Design review of the part built by this model. Coordinates are the model's own, in mm. Face numbers are marked on the shaded views. A direction names the side the tool comes from. Give positions to 0.01 mm unless a question says otherwise; leave off trailing zeros. Loops run counter-clockwise (first coordinate to the right, second up) from the corner with the lowest first, then second, coordinate; pieces in that order, holes last. Notation, with made-up numbers: (-10.75, 24) - (26.25, 24) arc R12 ccw to (26.25, 41) - close; hole circle Ø4 at (46.5, 75). An arc over 180 degrees is marked (long way). Write each question's results on one line, items separated by ' | '.
from build123d import *

# Parameters (mm, degrees)
BASE_DEPTH                = 7
SKETCH2_W                 = 9.8
SKETCH2_H                 = 13.6
PCB_CUTOUT_DEPTH          = 2.5
BASKET_WIRE_GROOVES_DEPTH = 30.49321956
SKETCH5_R                 = 1.4
SCREW_HOLES_DEPTH         = 28.14498112
F_1MM_EDGE_FILLETS_R      = 1


with BuildPart() as part:
    # Sketch1 → Base (new body)
    with BuildSketch(Plane(origin=(0, 0, 0), x_dir=(1, 0, 0), z_dir=(0, 1, 0))):
        Polygon((-8.9, 10.8), (-8.9, 5), (-23.9, 5), (-23.9, -5), (-8.9, -5), (-8.9, -10.8), (8.9, -10.8), (8.9, -5), (23.9, -5), (23.9, 5), (8.9, 5), (8.9, 10.8), (0, 10.8), align=None)
    extrude(amount=BASE_DEPTH)

    # Sketch2 → PCB Cutout (cut)
    with BuildSketch(Plane(origin=(0, 7, 0), x_dir=(1, 0, 0), z_dir=(0, 1, 0))):
        Rectangle(SKETCH2_W, SKETCH2_H)
    extrude(amount=-PCB_CUTOUT_DEPTH, mode=Mode.SUBTRACT)

    # Sketch4 → Basket Wire Grooves (cut, through all)
    with BuildSketch(Plane(origin=(0, 0, -5), x_dir=(-1, 0, 0), z_dir=(0, 0, -1))):
        with BuildLine():
            Line((-9.5, 0), (-15.5, 0))
            ThreePointArc((-15.5, 0), (-15.002081528, 1.202081528), (-13.8, 1.7))
            Line((-13.8, 1.7), (-11.2, 1.7))
            ThreePointArc((-11.2, 1.7), (-9.997918472, 1.202081528), (-9.5, 0))
        make_face()
        with BuildLine():
            Line((13.8, 1.7), (11.2, 1.7))
            ThreePointArc((11.2, 1.7), (9.997918472, 1.202081528), (9.5, 0))
            Line((9.5, 0), (15.5, 0))
            ThreePointArc((15.5, 0), (15.002081528, 1.202081528), (13.8, 1.7))
        make_face()
    extrude(amount=-BASKET_WIRE_GROOVES_DEPTH, mode=Mode.SUBTRACT)

    # Sketch5 → Screw Holes (cut, through all)
    with BuildSketch(Plane.XZ):
        with Locations(Location((-20.4, 0, 0), (0, 0, 270))):
            Circle(SKETCH5_R)
        with Locations(Location((20.4, 0, 0), (0, 0, 90))):
            Circle(SKETCH5_R)
    extrude(amount=-SCREW_HOLES_DEPTH, mode=Mode.SUBTRACT)

    # 1mm Edge Fillets
    # the kernel refuses this fillet: 1 mm, written as the material it adds along each edge
    with BuildSketch(Plane(origin=(8.9, 0, -5), x_dir=(0, 0, -1), z_dir=(0, 1, 0))) as f_1mm_edge_fillets_piece_1_section:
        with BuildLine():
            CenterArc((F_1MM_EDGE_FILLETS_R, -F_1MM_EDGE_FILLETS_R), F_1MM_EDGE_FILLETS_R, 90, 90)
            Line((0, -F_1MM_EDGE_FILLETS_R), (0, 0))
            Line((0, 0), (F_1MM_EDGE_FILLETS_R, 0))
        make_face()
    f_1mm_edge_fillets_piece_1 = extrude(amount=7, mode=Mode.PRIVATE)
    f_1mm_edge_fillets_piece_1 = f_1mm_edge_fillets_piece_1 - Plane(origin=(11.2, 0, -5.227855897), x_dir=(0, 1, 0), z_dir=(0, 0, -1)) * Cylinder(1.7, 18, mode=Mode.PRIVATE)
    add(f_1mm_edge_fillets_piece_1)
    with BuildSketch(Plane(origin=(8.9, 0, 5), x_dir=(1, 0, 0), z_dir=(0, 1, 0))) as f_1mm_edge_fillets_piece_2_section:
        with BuildLine():
            CenterArc((F_1MM_EDGE_FILLETS_R, -F_1MM_EDGE_FILLETS_R), F_1MM_EDGE_FILLETS_R, 90, 90)
            Line((0, -F_1MM_EDGE_FILLETS_R), (0, 0))
            Line((0, 0), (F_1MM_EDGE_FILLETS_R, 0))
        make_face()
    f_1mm_edge_fillets_piece_2 = extrude(amount=7, mode=Mode.PRIVATE)
    f_1mm_edge_fillets_piece_2 = f_1mm_edge_fillets_piece_2 - Plane(origin=(11.2, 0, 5.227855907), x_dir=(0, 1, 0), z_dir=(0, 0, -1)) * Cylinder(1.7, 19, mode=Mode.PRIVATE)
    add(f_1mm_edge_fillets_piece_2)
    with BuildSketch(Plane(origin=(-8.9, 0, 5), x_dir=(0, 0, 1), z_dir=(0, 1, 0))) as f_1mm_edge_fillets_piece_3_section:
        with BuildLine():
            CenterArc((F_1MM_EDGE_FILLETS_R, -F_1MM_EDGE_FILLETS_R), F_1MM_EDGE_FILLETS_R, 90, 90)
            Line((0, -F_1MM_EDGE_FILLETS_R), (0, 0))
            Line((0, 0), (F_1MM_EDGE_FILLETS_R, 0))
        make_face()
    f_1mm_edge_fillets_piece_3 = extrude(amount=7, mode=Mode.PRIVATE)
    f_1mm_edge_fillets_piece_3 = f_1mm_edge_fillets_piece_3 - Plane(origin=(-11.2, 0, 5.227855897), x_dir=(0, 1, 0), z_dir=(0, 0, -1)) * Cylinder(1.7, 18, mode=Mode.PRIVATE)
    add(f_1mm_edge_fillets_piece_3)
    with BuildSketch(Plane(origin=(-8.9, 0, -5), x_dir=(0, 0, -1), z_dir=(0, 1, 0))) as f_1mm_edge_fillets_piece_4_section:
        with BuildLine():
            CenterArc((F_1MM_EDGE_FILLETS_R, F_1MM_EDGE_FILLETS_R), F_1MM_EDGE_FILLETS_R, 180, 90)
            Line((0, F_1MM_EDGE_FILLETS_R), (0, 0))
            Line((0, 0), (F_1MM_EDGE_FILLETS_R, 0))
        make_face()
    f_1mm_edge_fillets_piece_4 = extrude(amount=7, mode=Mode.PRIVATE)
    f_1mm_edge_fillets_piece_4 = f_1mm_edge_fillets_piece_4 - Plane(origin=(-11.2, 0, -5.227855897), x_dir=(0, 1, 0), z_dir=(0, 0, -1)) * Cylinder(1.7, 19, mode=Mode.PRIVATE)
    add(f_1mm_edge_fillets_piece_4)
    # the kernel refuses this fillet: 1 mm, written as the material it takes off along each edge
    with BuildSketch(Plane(origin=(8.9, -2.5, -10.8), x_dir=(-1, 0, 0), z_dir=(0, 1, 0)), Plane(origin=(23.9, -2.5, -5), x_dir=(-1, 0, 0), z_dir=(0, 1, 0)), Plane(origin=(23.9, -2.5, 5), x_dir=(0, 0, -1), z_dir=(0, 1, 0)), Plane(origin=(8.9, -2.5, 10.8), x_dir=(0, 0, -1), z_dir=(0, 1, 0)), Plane(origin=(-8.9, -2.5, 10.8), x_dir=(1, 0, 0), z_dir=(0, 1, 0)), Plane(origin=(-23.9, -2.5, 5), x_dir=(1, 0, 0), z_dir=(0, 1, 0)), Plane(origin=(-23.9, -2.5, -5), x_dir=(0, 0, 1), z_dir=(0, 1, 0)), Plane(origin=(-8.9, -2.5, -10.8), x_dir=(0, 0, 1), z_dir=(0, 1, 0))) as f_1mm_edge_fillets_2_piece_1:
        with BuildLine():
            CenterArc((F_1MM_EDGE_FILLETS_R, F_1MM_EDGE_FILLETS_R), F_1MM_EDGE_FILLETS_R, 180, 90)
            Line((0, F_1MM_EDGE_FILLETS_R), (0, 0))
            Line((0, 0), (F_1MM_EDGE_FILLETS_R, 0))
        make_face()
    extrude(amount=12, mode=Mode.SUBTRACT)


solid = part.part
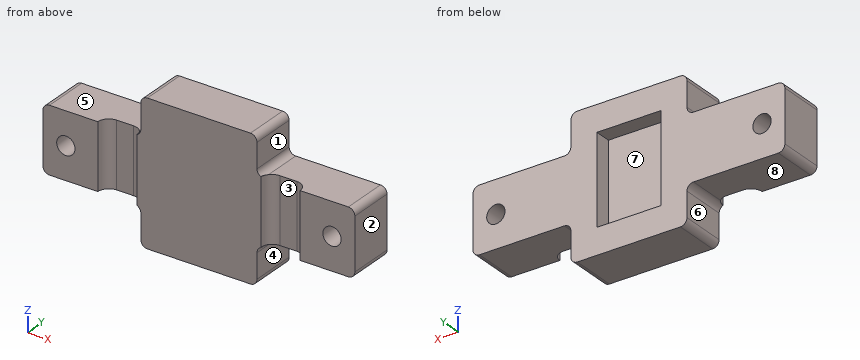
(1) Insertion check: P1, Ø1.1, axis at y = 2.5, z = 7.5, coming from the -X side; P2, Ø3, axis at y = 3, z = 8, coming from the +X side; P3, Ø3.5, axis at x = -14.5, y = 3, coming from the +Z side. Each pin has a flat end and moves straight along its axis. Give the tip position at first contact, or say it passes through.
Answers below:
P1: x = -8.9 | P2: x = 8.9 | P3: z = 5
(2) Wall thickness on line 1 along X through (y, z) = (5, 0); line 2 along X through (y, z) = (2, 0); line 3 along Z through (x, y) = (20.4, 2.25): over which ranges is each line inside the solid? List them lowest first. Write a range as from..to.
Answers below:
line 1: -23.9..-21.8, -19..-4.9, 4.9..19, 21.8..23.9 | line 2: -23.9..-21.8, -19..19, 21.8..23.9 | line 3: -5..-1.4, 1.4..5
(3) Draft analysis for pull direction Z (two halves, no side actions). For the marked faces 5, 6, 7 and 8, state which applies: pulls with the +Z half, pulls with the -Z half, needs draft (parallel to the pull), parting line crosses it, or undercut.
Answers below:
face 5: pulls with the +Z half | face 6: needs draft | face 7: undercut | face 8: pulls with the -Z half
(4) Take a section at C-C on y = 3. Give the boundary of the cut face in (x, z).
Answers below:
outline: (-23.9, -4) arc R1 ccw to (-22.9, -5) - (-9.9, -5) arc R1 cw to (-8.9, -6) - (-8.9, -9.8) arc R1 ccw to (-7.9, -10.8) - (7.9, -10.8) arc R1 ccw to (8.9, -9.8) - (8.9, -6) arc R1 cw to (9.9, -5) - (22.9, -5) arc R1 ccw to (23.9, -4) - (23.9, 4) arc R1 ccw to (22.9, 5) - (9.9, 5) arc R1 cw to (8.9, 6) - (8.9, 9.8) arc R1 ccw to (7.9, 10.8) - (-7.9, 10.8) arc R1 ccw to (-8.9, 9.8) - (-8.9, 6) arc R1 cw to (-9.9, 5) - (-22.9, 5) arc R1 ccw to (-23.9, 4) - close; hole circle Ø2.8 at (-20.4, 0); hole circle Ø2.8 at (20.4, 0)
(5) Take a section at B-B on x = 20.4. Give the boundary of the cut face in (y, z), plus the area to 3 significant figures.
Answers below:
outline: (0, -5) - (7, -5) - (7, -1.4) - (0, -1.4) - close; (0, 1.4) - (7, 1.4) - (7, 5) - (0, 5) - close | area: 50.4 mm2
(6) Tool access review of the marked faces 1, 2, 3 and 4: name each direction out of +Z, -Z, +X, -X, +Y, -Y from which nothing blocks a thin tool from reaching the whole face with its end or side.
Answers below:
face 1: +Z, +X, +Y, -Y | face 2: +Z, -Z, +X, +Y, -Y | face 3: +Z, -Z, -Y | face 4: -Z, +X, +Y, -Y
(7) Take a section at A-A on z = 0. Give the boundary of the cut face in (x, y).
Answers below:
outline: (-23.9, 0) - (-21.8, 0) - (-21.8, 7) - (-23.9, 7) - close; (-19, 0) - (-15.5, 0) arc R1.7 cw to (-13.8, 1.7) - (-11.2, 1.7) arc R1.7 cw to (-9.5, 0) - (9.5, 0) arc R1.7 cw to (11.2, 1.7) - (13.8, 1.7) arc R1.7 cw to (15.5, 0) - (19, 0) - (19, 7) - (4.9, 7) - (4.9, 4.5) - (-4.9, 4.5) - (-4.9, 7) - (-19, 7) - close; (21.8, 0) - (23.9, 0) - (23.9, 7) - (21.8, 7) - close
(8) Take a section at D-D on x = -3. Give the boundary of the cut face in (y, z), plus the area to 3 significant figures.
Answers below:
outline: (0, -10.8) - (7, -10.8) - (7, -6.8) - (4.5, -6.8) - (4.5, 6.8) - (7, 6.8) - (7, 10.8) - (0, 10.8) - close | area: 117 mm2
